Model file for the job. Use its own axes, mm. Face numbers are marked on the shaded views. A direction names the side the tool comes from. Give positions to 0.01 mm unless a question says otherwise; leave off trailing zeros. Write each loop counter-clockwise with the first axis right and the second up, starting at its lowest first coordinate (ties: lowest second). Pieces come first, ordered by that corner, then holes.
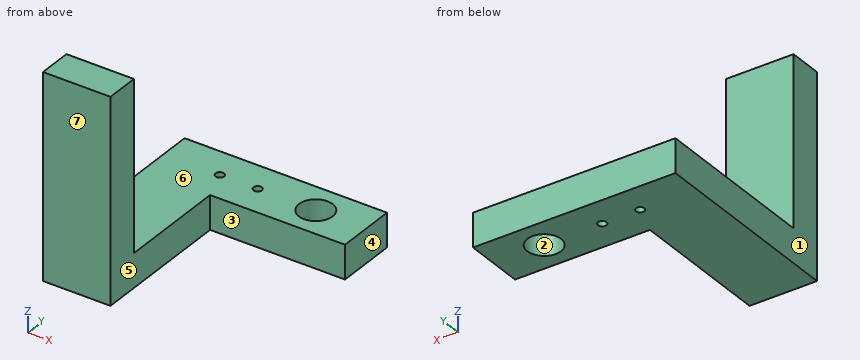
```python
from build123d import *

# Parameters (mm, degrees)
BOSS_EXTRUDE1_DEPTH = 5.08
SKETCH4_W           = 10.16
SKETCH4_H           = 5.08
BOSS_EXTRUDE2_DEPTH = 25.4
SKETCH2_R           = 0.635
SKETCH2_R_2         = 2.54
CUT_EXTRUDE1_DEPTH  = 5.08


with BuildPart() as part:
    # Sketch1 → Boss-Extrude1 (new body)
    with BuildSketch(Plane.XY):
        Polygon((-22.92, -4.55), (-22.92, -26.14), (-12.76, -26.14), (-12.76, -4.55), (7.56, -4.55), (7.56, 4.55), (-22.92, 4.55), align=None)
    extrude(amount=BOSS_EXTRUDE1_DEPTH)

    # Sketch4 → Boss-Extrude2 (add)
    with BuildSketch(Plane.XY.offset(5.08)):
        with Locations((-17.84, -23.6)):
            Rectangle(SKETCH4_W, SKETCH4_H)
    extrude(amount=BOSS_EXTRUDE2_DEPTH)

    # Sketch2 → Cut-Extrude1 (cut)
    with BuildSketch(Plane(origin=(0, 0, 0), x_dir=(-1, 0, 0), z_dir=(0, 0, -1))):
        with Locations((14.45, 0)):
            Circle(SKETCH2_R)
        Circle(SKETCH2_R_2)
        with Locations((8.75, 0)):
            Circle(SKETCH2_R)
    extrude(amount=-CUT_EXTRUDE1_DEPTH, mode=Mode.SUBTRACT)


solid = part.part
```
1. Slice it at D-D, the plane z = 15. Write the cut outline in (x, y).
Calculated:
outline: (-22.92, -26.14) - (-12.76, -26.14) - (-12.76, -21.06) - (-22.92, -21.06) - close
2. Probe probe 1 along Y at (x, z) = (0, 3.85); probe 2 along Y at (x, z) = (-19, 14); probe 3 along Z at (x, y) = (-20, 0). List the from-to ranges inside material, lowest first.
Calculated:
probe 1: y = -4.55 to -2.54, 2.54 to 4.55
probe 2: y = -26.14 to -21.06
probe 3: z = 0 to 5.08
3. Pull direction X, two halves, no side cores. Call the marked faces 1, 2, 3 and 4: +X half, -X half, draft (parallel to the pull), parting line (faces both ways), or undercut.
Calculated:
face 1: -X half
face 2: undercut
face 3: draft
face 4: +X half
4. Slice it at B-B, the plane y = 0. Write the cut outline in (x, z) (3 decimals), and give its area (3 significant figures).
Calculated:
outline: (-22.92, 0) - (-15.085, 0) - (-15.085, 5.08) - (-22.92, 5.08) - close; (-13.815, 0) - (-9.385, 0) - (-9.385, 5.08) - (-13.815, 5.08) - close; (-8.115, 0) - (-2.54, 0) - (-2.54, 5.08) - (-8.115, 5.08) - close; (2.54, 0) - (7.56, 0) - (7.56, 5.08) - (2.54, 5.08) - close
area: 116 mm2
5. Slice it at C-C, the plane x = -8.75. Write the cut outline in (y, z) (3 decimals), and give its area (3 significant figures).
Calculated:
outline: (-4.55, 0) - (-0.635, 0) - (-0.635, 5.08) - (-4.55, 5.08) - close; (0.635, 0) - (4.55, 0) - (4.55, 5.08) - (0.635, 5.08) - close
area: 39.8 mm2
6. Which spindle directions (+Z, -Z, +X, -X, +Y, -Y) get a long thin tool onto all of the face, cutting with end or side? Do the marked faces 5, 6 and 7. Say none if no direction does.
Calculated:
face 5: +Z, -Z, +X, -Y
face 6: +Z, +X, -X, +Y
face 7: +Z, -Z, +X, -X, -Y
7. Slice it at A-A, the plane x = -14.45. Write the cut outline in (y, z) (3 decimals).
Calculated:
outline: (-26.14, 0) - (-0.635, 0) - (-0.635, 5.08) - (-21.06, 5.08) - (-21.06, 30.48) - (-26.14, 30.48) - close; (0.635, 0) - (4.55, 0) - (4.55, 5.08) - (0.635, 5.08) - close
8. Pin check, flat tips, straight feed: P1, Ø7.5, axis at x = -6, y = -12.5, coming from the +Z side; P2, Ø12, axis at x = -2, z = 9.5, coming from the -Y side; P3, Ø6, axis at x = -18.5, y = -16, coming from the -Z side; P4, Ø8, axis at x = -18, z = 16, coming from the +Y side. Stop position of each tip, or through.
Calculated:
P1: passes through
P2: stops at y = -4.55
P3: stops at z = 0
P4: stops at y = -21.06
